Answer from the drawing. Dimensions are ordinates in mm from the lowest x, y and z of the part. Round coordinates to 2 decimals unless told otherwise and drop trailing zeros. Loops run counter-clockwise (first coordinate to the right, second up) from the corner with the lowest first, then second, coordinate; pieces in that order, holes last. Notation, with made-up numbers: (-10, 74) - (29, 74) arc R20 ccw to (29, 109) - close; hole circle Ø7 at (-9.5, 9). An arc over 180 degrees is marked (long way). Answer as CSV lines item,"result". Start each with the question number.
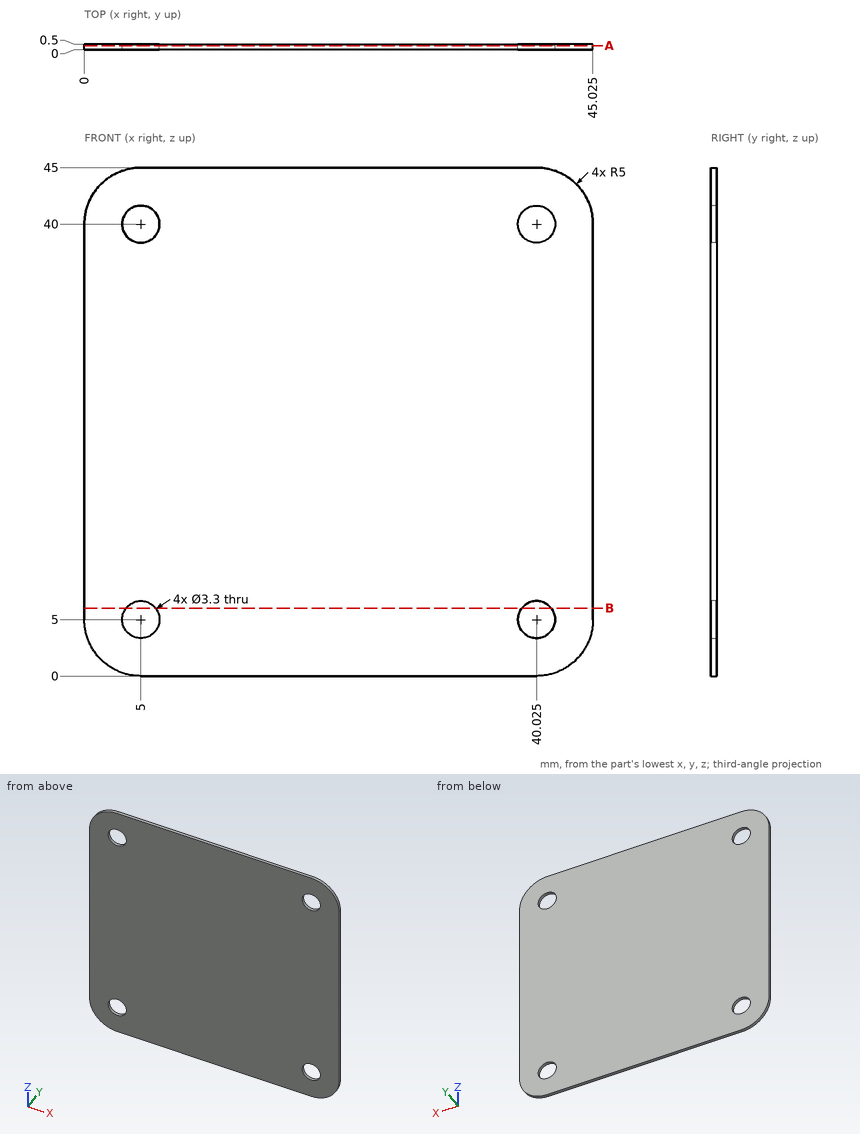
Item 1: Section A-A, the plane y = 0.35 is taken. Count the separate pieces of the cut face and the enclosed holes in it, and give its area (3 significant figures).
Item 2: Find the intervals of material crossed by L1, parallel to Z at x = 40, y = 0.1; L2, parallel to X at y = 0.3, z = 42; L3, parallel to Z at x = 42.5, y = 0.2 (1 decimal), in increasing order.
Item 3: A flat-ended cylindrical pin translates along its axis: pin 1 Ø5.5 at (x, z) = (5, 40) entering from -Y. Find the tip coordinate at first contact, or state that the pin passes through.
Item 4: Section B-B, the plane z = 6 is taken. Give the vertices of the cut face in (x, y) (1 decimal).
Answer:
1,separate pieces,"1"
1,enclosed holes,"4"
1,area,"1,970 mm²"
2,L1,"z = 0 to 3.35, 6.65 to 38.35, 41.65 to 45"
2,L2,"x = 0.42 to 44.61"
2,L3,"z = 0.7 to 44.3"
3,pin 1,"stops at y = 0"
4,outline,"(0, 0) - (3.7, 0) - (3.7, 0.5) - (0, 0.5) - close; (6.3, 0) - (38.7, 0) - (38.7, 0.5) - (6.3, 0.5) - close; (41.3, 0) - (45, 0) - (45, 0.5) - (41.3, 0.5) - close"
